The listing builds one solid part. Answer for the finished solid, in the listing's coordinates (mm). A direction names the side the tool comes from. Coordinates: 2 decimals unless noted, no trailing zeros. Write each loop counter-clockwise with the first axis right and the second up, starting at its lowest first coordinate (ties: lowest second). Pieces come first, ordered by that corner, then holes. Notation, with made-up numbers: M -10,65.5 L 6,65.5 A13 cw 6,89.5 Z; hole C 51,26.25 d2. An arc over 180 degrees is marked long. Answer as CSV lines item,"result".
```python
from build123d import *

# Parameters (mm, degrees)
SKETCH1_W               = 34.7
SKETCH1_H               = 27
SKETCH1_R               = 1.6
BOSS_EXTRUDE1_DEPTH     = 25
SKETCH4_R               = 1.6
SKETCH4_R_2             = 5.25
BASE_EXTRUDE_DEPTH      = 45.847965394
SKETCH4_3_R             = 11.25
SKETCH4_3_R_2           = 5.25
SKETCH4_3_R_3           = 1.6
CUT_EXTRUDE3_DEPTH      = 5
BOSS_EXTRUDE5_DEPTH     = 34.7
CHAMFER3_SIZE           = 12.5
CHAMFER3_SIZE2          = 15
FILLET1_R               = 10
FILLET3_R               = 20
FILLET4_R               = 7.5
BOSS_EXTRUDE6_DEPTH     = 7.5
FILLET5_R               = 2
SKETCH13_R              = 3.25
CUT_EXTRUDE5_DEPTH      = 18.5
CHAMFER4_SIZE           = 15
FILLET11_R              = 10
FILLET12_R              = 25
FILLET13_R              = 5
CUT_EXTRUDE6_DEPTH      = 66.246417783
CUT_EXTRUDE6_DEPTH_BACK = 66.246417783


with BuildPart() as part:
    # Sketch1 → Boss-Extrude1 (new body)
    with BuildSketch(Plane.XY):
        Rectangle(SKETCH1_W, SKETCH1_H)
        with Locations((-7.5, -10)):
            Circle(SKETCH1_R, mode=Mode.SUBTRACT)
        with Locations(Location((7.5, -10, 0), (0, 0, 180))):
            Circle(SKETCH1_R, mode=Mode.SUBTRACT)
        with Locations((7.5, 10)):
            Circle(SKETCH1_R, mode=Mode.SUBTRACT)
        with Locations(Location((-7.5, 10, 0), (0, 0, 180))):
            Circle(SKETCH1_R, mode=Mode.SUBTRACT)
    extrude(amount=BOSS_EXTRUDE1_DEPTH)

    # Sketch4 → Base Extrude (cut, through all)
    with BuildSketch(Plane.ZY.offset(17.35)):
        with Locations((6.343145751, 5.656854249)):
            Circle(SKETCH4_R)
        with Locations((17.656854249, 5.656854249)):
            Circle(SKETCH4_R)
        with Locations((17.656854249, -5.656854249)):
            Circle(SKETCH4_R)
        with Locations((6.343145751, -5.656854249)):
            Circle(SKETCH4_R)
        with Locations((12, 0)):
            Circle(SKETCH4_R_2)
    extrude(amount=-BASE_EXTRUDE_DEPTH, mode=Mode.SUBTRACT)

    # Sketch4<3> → Cut-Extrude3 (cut)
    with BuildSketch(Plane.ZY.offset(17.35)):
        with Locations((12, 0)):
            Circle(SKETCH4_3_R)
        with Locations((12, 0)):
            Circle(SKETCH4_3_R_2, mode=Mode.SUBTRACT)
        with Locations((6.343145751, 5.656854249)):
            Circle(SKETCH4_3_R_3, mode=Mode.SUBTRACT)
        with Locations((17.656854249, 5.656854249)):
            Circle(SKETCH4_3_R_3, mode=Mode.SUBTRACT)
        with Locations((17.656854249, -5.656854249)):
            Circle(SKETCH4_3_R_3, mode=Mode.SUBTRACT)
        with Locations((6.343145751, -5.656854249)):
            Circle(SKETCH4_3_R_3, mode=Mode.SUBTRACT)
    extrude(amount=-CUT_EXTRUDE3_DEPTH, mode=Mode.SUBTRACT)

    # Sketch10 → Boss-Extrude5 (add)
    with BuildSketch(Plane(origin=(17.35, 0, 0), x_dir=(0, 0, -1), z_dir=(1, 0, 0))):
        Polygon((0, 13.5), (0, 25), (53.849999999, 25), (53.849999999, 32.5), (-25, 32.5), (-25, 13.5), align=None)
        Polygon((-25, -13.5), (-25, -32.5), (53.849999999, -32.5), (53.849999999, -25), (0, -25), (0, -13.5), align=None)
    extrude(amount=-BOSS_EXTRUDE5_DEPTH)

    # Chamfer3
    chamfer3_edges = [part.edges().sort_by_distance(p)[0] for p in [
        (0, 32.5, 25),
    ]]
    chamfer3_side = [part.faces().sort_by_distance(p)[0] for p in [
        (0, 0, 25),
    ]]
    chamfer(chamfer3_edges, length=CHAMFER3_SIZE, length2=CHAMFER3_SIZE2, reference=chamfer3_side[0])

    # Fillet1
    fillet1_edges = [part.edges().sort_by_distance(p)[0] for p in [
        (0, 25, 0),
    ]]
    fillet(fillet1_edges, radius=FILLET1_R)

    # Fillet3
    fillet3_edges = [part.edges().sort_by_distance(p)[0] for p in [
        (0, 32.5, 10),
    ]]
    fillet(fillet3_edges, radius=FILLET3_R)

    # Fillet4
    fillet4_edges = [part.edges().sort_by_distance(p)[0] for p in [
        (0, 20, 25),
    ]]
    fillet(fillet4_edges, radius=FILLET4_R)

    # Sketch11 → Boss-Extrude6 (add)
    with BuildSketch(Plane.XZ.offset(-25)):
        with BuildLine():
            Line((-12, -53.849999999), (-17.35, -53.849999999))
            Line((-17.35, -53.849999999), (-17.35, -41.849999999))
            ThreePointArc((-17.35, -41.849999999), (0, -24.499999999), (17.35, -41.849999999))
            Line((17.35, -41.849999999), (17.35, -53.849999999))
            Line((17.35, -53.849999999), (12, -53.849999999))
            Line((12, -53.849999999), (12, -41.849999999))
            ThreePointArc((12, -41.849999999), (0, -29.849999999), (-12, -41.849999999))
            Line((-12, -41.849999999), (-12, -53.849999999))
        make_face()
    extrude(amount=BOSS_EXTRUDE6_DEPTH)

    # Fillet5
    # the kernel refuses this fillet: 2 mm, written as the material it adds along each edge
    with BuildSketch(Plane(origin=(0, 25, -41.849999999), x_dir=(-0.9586337455117862, 0, -0.28464248095820854), z_dir=(0.28464248095820854, 0, -0.9586337455117862))) as fillet5_piece_1_section:
        with BuildLine():
            CenterArc((19.3499, -1.9999), FILLET5_R, 90, 90)
            Line((17.3499, -1.9999), (17.3099, -1.9999))
            ThreePointArc((17.3099, -1.9999), (17.31, -0.99995), (17.31, 0))
            Line((17.31, 0), (17.35, 0.04))
            ThreePointArc((17.35, 0.04), (18.34995, 0.04), (19.3499, 0.0401))
            Line((19.3499, 0.0401), (19.3499, 0.0001))
        make_face()
    fillet5_piece_1 = revolve(axis=Axis((0, 25, -41.849999999), (0, 1, 0)), revolution_arc=213.074958292, mode=Mode.PRIVATE)
    fillet5_piece_1 = split(fillet5_piece_1, bisect_by=Plane(origin=(17.35, 24.441377489, -23.941377488), z_dir=(-1, 0, 0)), keep=Keep.TOP, mode=Mode.PRIVATE)
    fillet5_piece_1 = split(fillet5_piece_1, bisect_by=Plane(origin=(-17.35, 24.441377489, -23.941377488), z_dir=(1, 0, 0)), keep=Keep.TOP, mode=Mode.PRIVATE)
    add(fillet5_piece_1)

    # Sketch13 → Cut-Extrude5 (cut)
    with BuildSketch(Plane.XZ.offset(-25)):
        with Locations(Location((0, -41.849999999, 0), (0, 0, 270))):
            Circle(SKETCH13_R)
    extrude(amount=-CUT_EXTRUDE5_DEPTH, mode=Mode.SUBTRACT)

    # Mirror12: part across plane


with BuildPart() as part_1:
    add(part.part)
    add(part.part.mirror(Plane.ZX))

    # Chamfer4
    chamfer4_edges = [part_1.edges().sort_by_distance(p)[0] for p in [
        (0, 32.5, 25),
        (0, -32.5, 25),
    ]]
    chamfer(chamfer4_edges, length=CHAMFER4_SIZE)

    # Fillet11
    fillet11_edges = [part_1.edges().sort_by_distance(p)[0] for p in [
        (0, 17.5, 25),
        (0, -17.5, 25),
    ]]
    fillet(fillet11_edges, radius=FILLET11_R)

    # Fillet12
    fillet12_edges = [part_1.edges().sort_by_distance(p)[0] for p in [
        (0, -32.5, 10),
        (0, 32.5, 10),
    ]]
    fillet(fillet12_edges, radius=FILLET12_R)

    # Fillet13
    fillet13_edges = [part_1.edges().sort_by_distance(p)[0] for p in [
        (0, 32.5, -53.849999999),
        (0, -32.5, -53.849999999),
    ]]
    fillet(fillet13_edges, radius=FILLET13_R)

    # Sketch14 → Cut-Extrude6 (cut, two sides: drawn at the far end of the back side and taken through both)
    with BuildSketch(Plane(origin=(0, 0, 0), x_dir=(1, 0, 0), z_dir=(0, 1, 0)).offset(-CUT_EXTRUDE6_DEPTH_BACK)):
        with BuildLine():
            Line((-3.25, 40.849999999), (-3.25, 42.849999999))
            ThreePointArc((-3.25, 42.849999999), (0, 46.099999999), (3.25, 42.849999999))
            Line((3.25, 42.849999999), (3.25, 40.849999999))
            ThreePointArc((3.25, 40.849999999), (0, 37.599999999), (-3.25, 40.849999999))
        make_face()
    extrude(amount=CUT_EXTRUDE6_DEPTH + CUT_EXTRUDE6_DEPTH_BACK, mode=Mode.SUBTRACT)


solid = part_1.part
```
Q1. Flat-ended cylindrical pins translate along their axes: pin 1 Ø8 at (x, y) = (2.5, 19.5) entering from +Z; pin 2 Ø1.5 at (x, y) = (-3, -0.5) entering from -Z; pin 3 Ø1.9 at (y, z) = (-5.66, 6.34) entering from -X; pin 4 Ø1 at (x, y) = (3, -23) entering from -Z. Find the tip coordinate at first contact, or state that the pin passes through.
Output:
pin 1,"z = 24.77"
pin 2,"z = 0"
pin 3,"through"
pin 4,"z = -30.37"
Q2. The mould has two halves that part along Y. Classify faces 1 (the flat face through (0, 26, -53.85)), 2 (the flat face through (-12, -21, -48)), 3 (the flat face through (0.2, 22.8, 19.7)): pulls with the +Y half, pulls with the -Y half, needs draft (parallel to the pull), parting line crosses it, or undercut.
Output:
face 1,"needs draft"
face 2,"undercut"
face 3,"pulls with the +Y half"
Q3. Find section A-A (z = -11). Give the vertices of the cut face in (x, y), and give its area (4 significant figures).
Output:
outline,"M -17.35,-32.5 L 17.35,-32.5 L 17.35,-25 L -17.35,-25 Z; M -17.35,25 L 17.35,25 L 17.35,32.5 L -17.35,32.5 Z"
area,"520.5 mm2"
Q4. Find section B-B (x = 0). Count the separate pieces of the cut face and the enclosed holes in it, and give its area (3 significant figures).
Output:
separate pieces,"3"
enclosed holes,"5"
area,"2,040 mm2"
Q5. Find section D-D (z = 20.5). Give the vertices of the cut face in (x, y).
Output:
outline,"M -17.35,-22 L 17.35,-22 L 17.35,22 L -17.35,22 L -17.35,7.37 L -12.35,7.37 L -12.35,-7.37 L -17.35,-7.37 Z; hole C -7.5,-10 d3.2; hole C -7.5,10 d3.2; hole C 7.5,-10 d3.2; hole C 7.5,10 d3.2"
Q6. Find section C-C (y = -10). Give the vertices of the cut face in (x, z).
Output:
outline,"M -17.35,0 L -9.1,0 L -9.1,25 L -17.35,25 L -17.35,17.15 L -12.35,17.15 L -12.35,6.85 L -17.35,6.85 Z; M -5.9,0 L 5.9,0 L 5.9,25 L -5.9,25 Z; M 9.1,0 L 17.35,0 L 17.35,25 L 9.1,25 Z"
Q7. For faces 4 (the cylindrical face through (-0.24, -22.15, -3.01)), 5 (the flat face through (-12, 21, -48)), 6 (the flat face through (-3.25, -29, -42)), determine the directions among +Z, -Z, +X, -X, +Y, -Y from which every point of the face is accessible in a straight line to the end or side of a thin tool.
Output:
face 4,"+X, -X"
face 5,"-Z"
face 6,"+Y, -Y"
Q8. Straight lines are drawn through the part: line 1 (X direction, y = -10, z = 13.75); line 2 (X direction, y = 10, z = 5); line 3 (X direction, y = 20, z = -43). For each, find the intervals that lie inside material, in ascending order.
Output:
line 1,"-12.35 to -9.1, -5.9 to 5.9, 9.1 to 17.35"
line 2,"-17.35 to -9.1, -5.9 to 5.9, 9.1 to 17.35"
line 3,"-17.35 to -12, 12 to 17.35"
